Design review of the part built by this model. Coordinates are the model's own, in mm. Give positions to 0.01 mm unless a question says otherwise; leave off trailing zeros. Loops run counter-clockwise (first coordinate to the right, second up) from the corner with the lowest first, then second, coordinate; pieces in that order, holes last. Notation, with made-up numbers: (36, 1.25) - (93, 1.25) arc R36 cw to (93, 36.25) - close; hole circle Ø6 at (-23, -25). An arc over 180 degrees is marked (long way). Write each question's results on one line, items separated by ' | '.
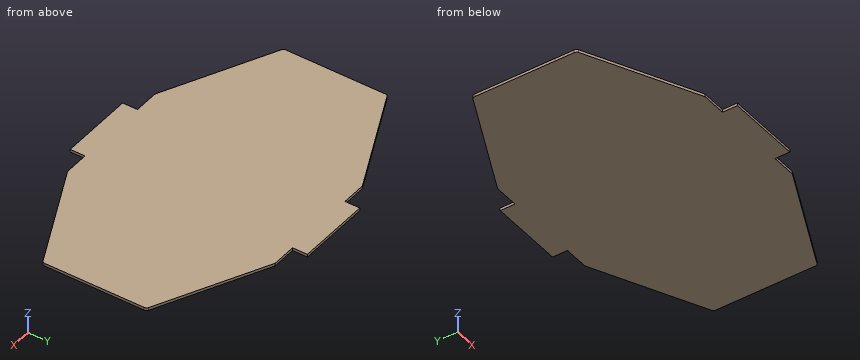
Autodesk Inventor part; units mm, degrees
ref_plane "Work Plane1" through (220.2461, -195.2123, 0) normal (0, -1, 0) x (1, 0, 0)
ref_plane "YZ Plane" through (0, 0, 0) normal (1, 0, 0) x (0, 1, 0)
ref_plane "XZ Plane" through (0, 0, 0) normal (0, 1, 0) x (-1, 0, 0)
sketch "Sketch1" plane through (0, 0, 0) normal (0, 0, 1) x (1, 0, 0)
  line L0 (42.4461, -373.0123) -> (525.0461, -373.0123)
  line L1 (575.8461, -322.2123) -> (575.8461, -68.2123) construction
  line L2 (525.0461, -17.4123) -> (42.4461, -17.4123)
  line L3 (-8.3539, -68.2123) -> (-8.3539, -322.2123) construction
  arc A0 (575.8461, -68.2123) -> (525.0461, -17.4123) centre (525.0461, -68.2123) ccw
  arc A1 (525.0461, -373.0123) -> (575.8461, -322.2123) centre (525.0461, -322.2123) ccw
  arc A2 (-8.3539, -322.2123) -> (42.4461, -373.0123) centre (42.4461, -322.2123) ccw
  arc A3 (42.4461, -17.4123) -> (-8.3539, -68.2123) centre (42.4461, -68.2123) ccw
  line L4 (-8.3539, -195.2123) -> (575.8461, -195.2123) construction
  line L5 (-8.3539, -106.3123) -> (177.9452, -17.4123)
  line L6 (-8.3539, -106.3123) -> (198.0693, -106.3123) construction
  line L7 (-8.3539, -284.1123) -> (177.9452, -373.0123)
  line L8 (283.7461, -17.4123) -> (283.7461, -373.0123) construction
  line L9 (575.8461, -106.3123) -> (389.5471, -17.4123)
  line L10 (575.8461, -284.1123) -> (389.5471, -373.0123)
  line L11 (575.8461, -106.3123) -> (575.8461, -284.1123)
  line L12 (-8.3539, -106.3123) -> (-8.3539, -284.1123)
  line L13 (177.9452, -17.4123) -> (389.5471, -17.4123)
  line L14 (389.5471, -373.0123) -> (177.9452, -373.0123)
  point P0 (0, 0)
  point P1 (-8.3539, -373.0123)
  point P2 (575.8461, -17.4123)
  point P3 (575.8461, -373.0123)
  point P4 (-8.3539, -17.4123)
  dimension "d0" = 355.6
  dimension "d1" = 584.2
  dimension "d4" = 50.8
  dimension "d25" = 25.51
  dimension "d26" = 254
  dimension "d27" = 88.9
  dimension "d28" = 575.8461
  dimension "d29" = 195.2123
extrude "Extrusion1" add sketch "Sketch1" along normal blind 4.7625
sketch "Sketch2" plane through (0, 0, 0) normal (0, 0, 1) x (1, 0, 0)
  line L0 (283.7461, -373.0123) -> (347.2461, -373.0123)
  line L1 (347.2461, -373.0123) -> (347.2461, -398.4123)
  line L2 (347.2461, -398.4123) -> (283.7461, -398.4123)
  line L3 (220.2461, -373.0123) -> (347.2461, -373.0123)
  line L4 (347.2461, -373.0123) -> (347.2461, -398.4123)
  line L5 (347.2461, -398.4123) -> (220.2461, -398.4123)
  line L6 (220.2461, -398.4123) -> (220.2461, -373.0123)
  line L7 (220.2461, -373.0123) -> (347.2461, -398.4123) construction
  line L8 (347.2461, -373.0123) -> (220.2461, -398.4123) construction
  line L9 (283.7461, -17.4123) -> (347.2461, -17.4123)
  line L10 (347.2461, -17.4123) -> (347.2461, 7.9877)
  line L11 (347.2461, 7.9877) -> (283.7461, 7.9877)
  line L12 (220.2461, -17.4123) -> (347.2461, -17.4123)
  line L13 (347.2461, -17.4123) -> (347.2461, 7.9877)
  line L14 (347.2461, 7.9877) -> (220.2461, 7.9877)
  line L15 (220.2461, 7.9877) -> (220.2461, -17.4123)
  line L16 (220.2461, -17.4123) -> (347.2461, 7.9877) construction
  line L17 (347.2461, -17.4123) -> (220.2461, 7.9877) construction
extrude "Extrusion2" add sketch "Sketch2" along normal up to surface (4.7625 mm away)
fillet "Fillet1" radius 6 8 edges at (-8.3539, -106.3123, 2.3813) (-8.3539, -284.1123, 2.3813) (177.9452, -373.0123, 2.3813) (389.5471, -373.0123, 2.3813) (575.8461, -284.1123, 2.3813) (575.8461, -106.3123, 2.3813) (389.5471, -17.4123, 2.3813) (177.9452, -17.4123, 2.3813)
ref_plane "Work Plane1" through (220.2461, -195.2123, 0) normal (0, -1, 0) x (1, 0, 0)
ref_plane "Work Plane2" through (283.7461, -280.3273, 0) normal (1, 0, 0) x (0, 0, -1)
properties part number "1211_Racetrack Board_V1" material "GFRP"
Item 1: We need section A-A on z = 1. Give the boundary of the cut face in (x, y), then the cut area to 3 significant figures.
Output values:
outline: (-8.35, -280.33) arc R6 ccw to (-4.94, -285.74) - (176.72, -372.43) arc R6 ccw to (179.3, -373.01) - (220.25, -373.01) - (220.25, -398.41) - (347.25, -398.41) - (347.25, -373.01) - (388.19, -373.01) arc R6 ccw to (390.77, -372.43) - (572.43, -285.74) arc R6 ccw to (575.85, -280.33) - (575.85, -110.1) arc R6 ccw to (572.43, -104.68) - (390.77, -18) arc R6 ccw to (388.19, -17.41) - (347.25, -17.41) - (347.25, 7.99) - (220.25, 7.99) - (220.25, -17.41) - (179.3, -17.41) arc R6 ccw to (176.72, -18) - (-4.94, -104.68) arc R6 ccw to (-8.35, -110.1) - close | area: 181,000 mm²
Item 2: Wall thickness on probe 1 along X at (y, z) = (-375, 0.8); probe 2 along Y at (x, z) = (368, 0.85); probe 3 along X at (y, z) = (-313.5, 0.55): over which ranges is each line inside the solid? List them lowest first.
Output values:
probe 1: x = 220.25 to 347.25 | probe 2: y = -373.01 to -17.41 | probe 3: x = 53.23 to 514.26
Item 3: We need section B-B on x = 214. Give the boundary of the cut face in (y, z).
Output values:
outline: (-373.01, 0) - (-17.41, 0) - (-17.41, 4.76) - (-373.01, 4.76) - close
Item 4: We need section C-C on y = -341. Give the boundary of the cut face in (x, z).
Output values:
outline: (110.86, 0) - (456.63, 0) - (456.63, 4.76) - (110.86, 4.76) - close
Item 5: Clearance check with flat-ended pins moving along their axes: P1, Ø1.4, axis at y = -6, z = 3, coming from the +X side; P2, Ø2.5, axis at x = 359, z = 2, coming from the +Y side; P3, Ø2.5, axis at y = -1.5, z = 3.5, coming from the -X side. State where each tip first meets the part, or that it passes through.
Output values:
P1: stops at x = 347.25 | P2: stops at y = -17.41 | P3: stops at x = 220.25
